```python
from build123d import *

# Parameters (mm, degrees)
EXTRUDE_2_DEPTH     = 18
SHELL_3_T           = -2
SKETCH_2_W          = 14.4
SKETCH_2_H          = 11.6
CUT_EXTRUDE_1_DEPTH = 10
SKETCH_3_W          = 12.5
SKETCH_3_H          = 5
CUT_EXTRUDE_2_DEPTH = 10
SKETCH_4_R          = 22.5
EXTRUDE_5_DEPTH     = 7
SHELL_START         = 2
SHELL_4_OUTLINE_R   = 20.5
SHELL_4_DEPTH       = 7
SKETCH_6_W          = 9
SKETCH_6_H          = 6.786647167
CUT_EXTRUDE_4_DEPTH = 14
SKETCH_9_W          = 2
SKETCH_9_H          = 3.464226151
SKETCH_9_H_2        = 3.181171453
SKETCH_9_H_3        = 3.477296157
EXTRUDE_6_DEPTH     = 7
EXTRUDE_8_DEPTH     = 2
SKETCH_11_W         = 7
SKETCH_11_H         = 1
CUT_EXTRUDE_5_DEPTH = 2


# Read off the part's stored shape, not the designer's step: 抽壳4
with BuildPart() as part:
    # 草图1 → 凸台-拉伸2 (new body)
    with BuildSketch(Plane(origin=(0, 0, 0), x_dir=(1, 0, 0), z_dir=(0, 1, 0))):
        with BuildLine():
            Line((-99.99792574, 53.871425224), (150.00207426, 53.871425224))
            Line((150.00207426, 53.871425224), (150.00207426, -95.878574776))
            ThreePointArc((150.00207426, -95.878574776), (147.073142072, -102.949642588), (140.00207426, -105.878574776))
            Line((140.00207426, -105.878574776), (-89.99792574, -105.878574776))
            ThreePointArc((-89.99792574, -105.878574776), (-97.068993552, -102.949642588), (-99.99792574, -95.878574776))
            Line((-99.99792574, -95.878574776), (-99.99792574, 53.871425224))
        make_face()
    extrude(amount=EXTRUDE_2_DEPTH)

    # 抽壳3
    shell_3_openings = [part.faces().sort_by_distance(p)[0] for p in [
        (25.00207426, 18, 25.920044782),
    ]]
    offset(amount=SHELL_3_T, openings=shell_3_openings, kind=Kind.INTERSECTION)

    # 草图2 → 切除-拉伸1 (cut)
    with BuildSketch(Plane.XY.offset(-51.871425224)):
        with Locations((-85.29792574, 7.8)):
            Rectangle(SKETCH_2_W, SKETCH_2_H)
    extrude(amount=-CUT_EXTRUDE_1_DEPTH, mode=Mode.SUBTRACT)

    # 草图3 → 切除-拉伸2 (cut)
    with BuildSketch(Plane(origin=(-97.99792574, 0, 0), x_dir=(0, 0, -1), z_dir=(1, 0, 0))):
        with Locations((17.621425224, 8.7)):
            Rectangle(SKETCH_3_W, SKETCH_3_H)
        with Locations((-1.978574776, 8.7)):
            Rectangle(SKETCH_3_W, SKETCH_3_H)
        with Locations((-21.578574776, 8.7)):
            Rectangle(SKETCH_3_W, SKETCH_3_H)
    extrude(amount=-CUT_EXTRUDE_2_DEPTH, mode=Mode.SUBTRACT)

    # 草图4 → 凸台-拉伸5 (add)
    with BuildSketch(Plane(origin=(0, 2, 0), x_dir=(1, 0, 0), z_dir=(0, 1, 0))):
        with Locations(Location((-73.49792574, -79.378574776, 0), (0, 0, 90))):
            Circle(SKETCH_4_R)
        with Locations(Location((123.50207426, -79.378574776, 0), (0, 0, 90))):
            Circle(SKETCH_4_R)
    extrude(amount=EXTRUDE_5_DEPTH)

    # 抽壳4 outline → 抽壳4 (cut)
    with BuildSketch(Plane(origin=(0, 0, 0), x_dir=(1, 0, 0), z_dir=(0, 1, 0)).offset(SHELL_START)):
        with Locations((123.50207426, -79.378574776)):
            Circle(SHELL_4_OUTLINE_R)
        with Locations((-73.49792574, -79.378574776)):
            Circle(SHELL_4_OUTLINE_R)
    extrude(amount=SHELL_4_DEPTH, mode=Mode.SUBTRACT)

    # 草图6 → 切除-拉伸4 (cut)
    with BuildSketch(Plane(origin=(0, 2, 0), x_dir=(1, 0, 0), z_dir=(0, 1, 0))):
        with Locations((-73.49792574, -100.485251193)):
            Rectangle(SKETCH_6_W, SKETCH_6_H)
        with Locations((123.50207426, -100.485251193)):
            Rectangle(SKETCH_6_W, SKETCH_6_H)
    extrude(amount=CUT_EXTRUDE_4_DEPTH, mode=Mode.SUBTRACT)

    # 草图9 → 凸台-拉伸6 (add)
    with BuildSketch(Plane(origin=(0, 2, 0), x_dir=(1, 0, 0), z_dir=(0, 1, 0))):
        with Locations((-78.99792574, -102.1464617)):
            Rectangle(SKETCH_9_W, SKETCH_9_H)
        with Locations((-67.99792574, -102.287989049)):
            Rectangle(SKETCH_9_W, SKETCH_9_H_2)
        with Locations((129.00207426, -102.287989049)):
            Rectangle(SKETCH_9_W, SKETCH_9_H_2)
        with Locations((118.00207426, -102.139926698)):
            Rectangle(SKETCH_9_W, SKETCH_9_H_3)
    extrude(amount=EXTRUDE_6_DEPTH)

    # 草图10 → 凸台-拉伸8 (add)
    with BuildSketch(Plane(origin=(0, 2, 0), x_dir=(1, 0, 0), z_dir=(0, 1, 0))):
        with BuildLine():
            Line((-77.99792574, -99.378574776), (-77.99792574, -97.322933221))
            ThreePointArc((-77.99792574, -97.322933221), (-73.49792574, -60.878574776), (-68.99792574, -97.322933221))
            Line((-68.99792574, -97.322933221), (-68.99792574, -99.378574776))
            ThreePointArc((-68.99792574, -99.378574776), (-73.49792574, -58.878574776), (-77.99792574, -99.378574776))
        make_face()
        with BuildLine():
            Line((119.00207426, -97.322933221), (119.00207426, -99.378574776))
            ThreePointArc((119.00207426, -99.378574776), (123.50207426, -58.878574776), (128.00207426, -99.378574776))
            Line((128.00207426, -99.378574776), (128.00207426, -97.322933221))
            ThreePointArc((128.00207426, -97.322933221), (123.50207426, -60.878574776), (119.00207426, -97.322933221))
        make_face()
    extrude(amount=EXTRUDE_8_DEPTH)

    # 草图11 → 切除-拉伸5 (cut)
    with BuildSketch(Plane(origin=(0, 0, 103.878574776), x_dir=(-1, 0, 0), z_dir=(0, 0, -1))):
        with Locations((73.49792574, 2.5)):
            Rectangle(SKETCH_11_W, SKETCH_11_H)
        with Locations((-123.50207426, 2.5)):
            Rectangle(SKETCH_11_W, SKETCH_11_H)
    extrude(amount=-CUT_EXTRUDE_5_DEPTH, mode=Mode.SUBTRACT)


solid = part.part
```
For this review, take the finished solid that the model builds, in its own axes (mm). A direction names the side the tool comes from. Round coordinates to 2 decimals unless told otherwise and drop trailing zeros. Write each loop counter-clockwise with the first axis right and the second up, starting at its lowest first coordinate (ties: lowest second). Pieces come first, ordered by that corner, then holes. Notation, with made-up numbers: (-36, 75.25) -> (15, 75.25) arc R23 cw to (15, 96.25) -> close; hole circle Ø11 at (78.5, 76). An arc over 180 degrees is marked (long way). One line per question, with ' | ' between items. Start each with the question number.
1) Mouldability with a two-part tool opening along X and no side actions: class faces 3 (the cylindrical face through (-72.66, 6.465, 58.896)), 4 (the cylindrical face through (147.15, 8.87, 102.87)), 5 (the flat face through (-99.998, 13, 22)), 6 (the flat face through (23, 10, -51.871)) as +X half, -X half, draft (parallel to the pull), parting line (faces both ways), or undercut.
2) Add section C-C (z = 53). Write out the cut boundary in (x, y), and give its area (3 significant figures).
3) Add section D-D (x = -13.5). Write out the cut boundary in (y, z), and give its area (4 significant figures).
4) Add section B-B (x = -73.5). Write out the cut boundary in (y, z).
5) Machinability: for faces 1 (the flat face through (27, 10, 103.879)), 2 (the flat face through (27, 0, 25)), which of the approach directions +Z, -Z, +X, -X, +Y, -Y give a long, thin tool a straight path to every point of the face, cutting with its end or side? Answer none if there is none.
6) Add section A-A (z = 22). Write out the cut boundary in (x, y).
7) Wall thickness on line 1 along X through (y, z) = (11.25, 10.5); line 2 along Z through (x, y) = (-34, 5.75); line 3 along X through (y, z) = (4.25, 65.5): over which ranges is each line inside the solid? List them lowest first.
8) For pin 1 Ø1.6 at (x, y) = (-99, 9) entering from +Z; pin 2 Ø2 at (y, z) = (5, 99) entering from -X; pin 3 Ø7 at (y, z) = (4, 101.5) entering from +X, all flat-tipped, find the tip position at first contact; note any pin that passes through.
Reported:
1) face 3: undercut | face 4: +X half | face 5: -X half | face 6: undercut
2) outline: (-100, 0) -> (150, 0) -> (150, 18) -> (148, 18) -> (148, 2) -> (-98, 2) -> (-98, 18) -> (-100, 18) -> close | area: 564 mm²
3) outline: (0, -53.87) -> (18, -53.87) -> (18, -51.87) -> (2, -51.87) -> (2, 103.88) -> (18, 103.88) -> (18, 105.88) -> (0, 105.88) -> close | area: 383.5 mm²
4) outline: (0, -53.87) -> (18, -53.87) -> (18, -51.87) -> (2, -51.87) -> (2, 56.88) -> (9, 56.88) -> (9, 58.88) -> (4, 58.88) -> (4, 60.88) -> (2, 60.88) -> (2, 105.88) -> (0, 105.88) -> close; (3, 103.88) -> (18, 103.88) -> (18, 105.88) -> (3, 105.88) -> close
5) face 1: +Y | face 2: +Z, -Z, +X, -X, -Y
6) outline: (-100, 0) -> (150, 0) -> (150, 18) -> (148, 18) -> (148, 2) -> (-98, 2) -> (-98, 6.2) -> (-100, 6.2) -> close; (-100, 11.2) -> (-98, 11.2) -> (-98, 18) -> (-100, 18) -> close
7) line 1: x = -100 to -98, 148 to 150 | line 2: z = -53.87 to -51.87, 103.88 to 105.88 | line 3: x = -100 to -98, -91.21 to -88.59, -58.41 to -55.79, 105.79 to 108.41, 138.59 to 141.21, 148 to 150
8) pin 1: stops at z = 101.6 | pin 2: stops at x = -99.77 | pin 3: stops at x = 149.77
